Can you work these out from the drawing? Everything is in mm from the part's minimum corner. A direction names the side the tool comes from. Round coordinates to 2 decimals unless told otherwise and drop trailing zeros. Order: outer loops, then holes, each group sorted by start corner. A loop starts at its lowest first (then second) coordinate and runs counter-clockwise, first axis right, second up. Notation, with made-up numbers: (26.5, 41.25) -> (68.5, 41.25) arc R20 cw to (68.5, 62.25) -> close; hole circle Ø7 at (-3, -0.75). An arc over 180 degrees is marked (long way). One line per item, written item: value.
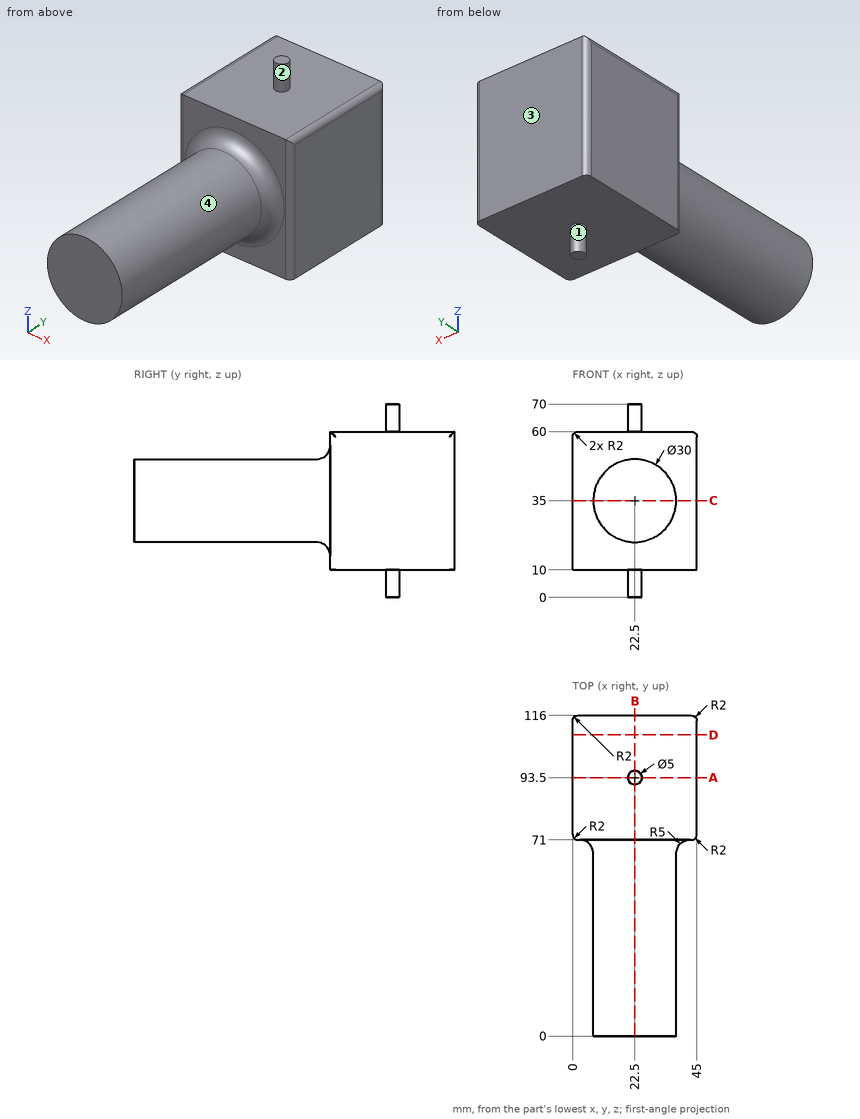
Q1. Please list where these lines run through material, in increasing order: line 1 along Y through (x, z) = (3.5, 42.5); line 2 along Z through (x, y) = (39, 100.5); line 3 along X through (y, z) = (27.5, 23).
Answers below:
line 1: 71 to 116
line 2: 10 to 60
line 3: 13.5 to 31.5
Q2. I want a section at A-A on y = 93.5. List the corners of the cut face in (x, z) for me, plus the area to 3 significant figures.
Answers below:
outline: (0, 10) -> (20, 10) -> (20, 0) -> (25, 0) -> (25, 10) -> (45, 10) -> (45, 58) arc R2 ccw to (43, 60) -> (25, 60) -> (25, 70) -> (20, 70) -> (20, 60) -> (2, 60) arc R2 ccw to (0, 58) -> close
area: 2,350 mm^2
Q3. I want a section at B-B on x = 22.5. List the corners of the cut face in (y, z) for me.
Answers below:
outline: (0, 20) -> (66, 20) arc R5 cw to (71, 15) -> (71, 10) -> (91, 10) -> (91, 0) -> (96, 0) -> (96, 10) -> (116, 10) -> (116, 60) -> (96, 60) -> (96, 70) -> (91, 70) -> (91, 60) -> (71, 60) -> (71, 55) arc R5 cw to (66, 50) -> (0, 50) -> close
Q4. On a 3-axis mill with a long thin cutter (end or side, diameter ignored), from which of +Z, -Z, +X, -X, +Y, -Y can I reach the whole of each face in a straight line? I mean the marked faces 1, 2, 3 and 4. Say none if no direction works.
Answers below:
face 1: -Z
face 2: +Z
face 3: +Z, -Z, +X, -X, +Y
face 4: -Y
Q5. I want a section at C-C on z = 35. List the corners of the cut face in (x, y) for me.
Answers below:
outline: (0, 73) arc R2 ccw to (2, 71) -> (2.5, 71) arc R5 cw to (7.5, 66) -> (7.5, 0) -> (37.5, 0) -> (37.5, 66) arc R5 cw to (42.5, 71) -> (43, 71) arc R2 ccw to (45, 73) -> (45, 114) arc R2 ccw to (43, 116) -> (2, 116) arc R2 ccw to (0, 114) -> close
Q6. Will these pins go through, and if not, where does the flat tip stop? pin 1 Ø8 at (x, z) = (18, 38) entering from -Y; pin 2 Ø6 at (y, z) = (34, 21.5) entering from +X; pin 3 Ø3 at (x, z) = (32, 60) entering from -Y.
Answers below:
pin 1: y = 0
pin 2: x = 33.21
pin 3: y = 71
Q7. I want a section at D-D on y = 109. List the corners of the cut face in (x, z) for me, plus the area to 3 significant figures.
Answers below:
outline: (0, 10) -> (45, 10) -> (45, 58) arc R2 ccw to (43, 60) -> (2, 60) arc R2 ccw to (0, 58) -> close
area: 2,250 mm^2
